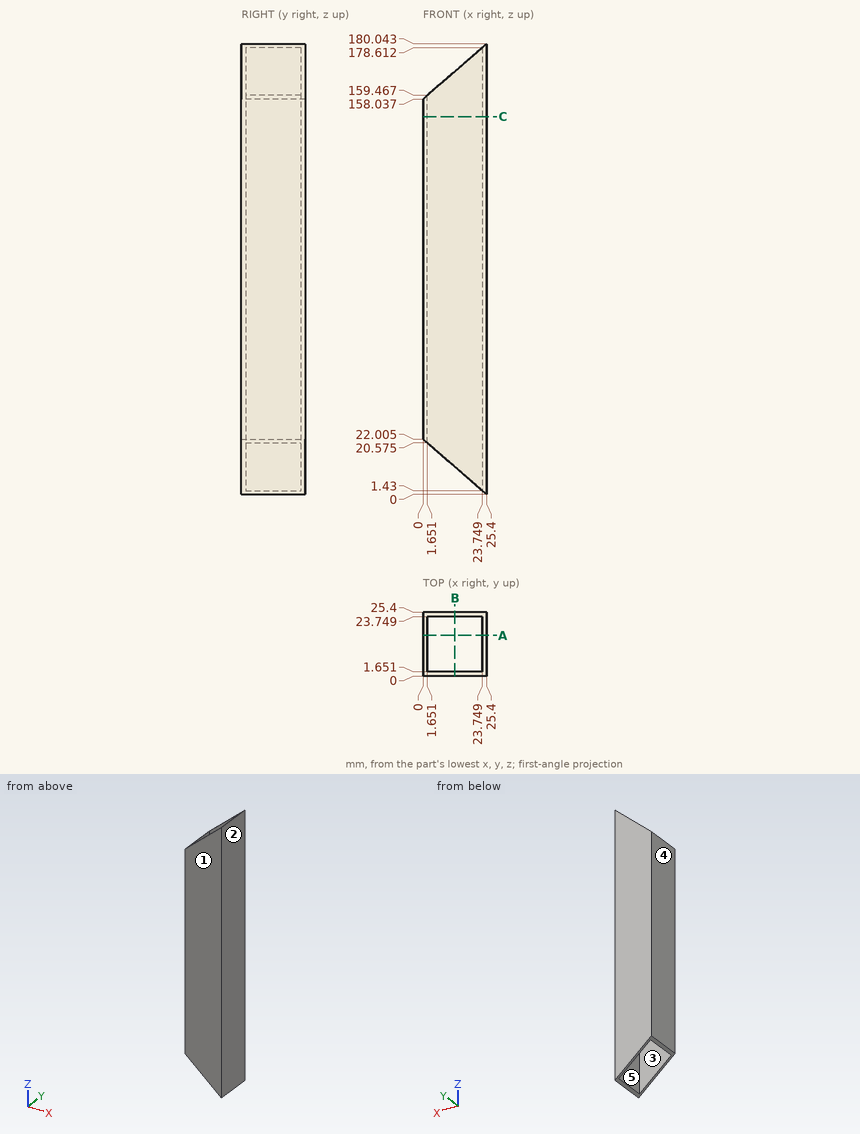
Study the drawing (mm; zero at the part's minimum x, y, z) and answer. A direction names the side the tool comes from. Round coordinates to 2 decimals unless told otherwise and drop trailing zeros. Write each loop counter-clockwise with the first axis right and the second up, starting at its lowest first coordinate (ties: lowest second). Pieces come first, ordered by that corner, then holes. Notation, with made-up numbers: (82, -30) -> (128, -30) arc R16 cw to (128, -10) -> close; hole circle Ø8 at (21, 53). An arc over 180 degrees is marked (long way). Answer as CSV lines item,"result". Start each with the question number.
(1) The part is cut by section C-C, the plane z = 151. Give the vertices of the cut face in (x, y).
(2) The part is cut by section A-A, the plane y = 16.25. Give the vertices of the cut face in (x, z) (1 decimal).
(3) A tool of negligible diameter and unlimited length cuts with its end or side. For the marked faces 4 and 5, from which of +Z, -Z, +X, -X, +Y, -Y can it reach the whole face along a straight path? Write none if from no direction.
(4) The part is cut by section B-B, the plane x = 12.75. Give the vertices of the cut face in (y, z).
(5) Find the intervals of material crossed by probe 1 along X at (y, z) = (22, 113); probe 2 along X at (y, z) = (15.75, 16), in increasing order.
(6) The mould has two halves that part along Y. Classify the marked faces 1, 2 and 3: +Y half, -Y half, draft (parallel to the pull), parting line (faces both ways), or undercut.
Output values:
1,outline,"(0, 0) -> (25.4, 0) -> (25.4, 25.4) -> (0, 25.4) -> close; hole (1.65, 1.65) -> (23.75, 1.65) -> (23.75, 23.75) -> (1.65, 23.75) -> close"
2,outline,"(0, 22) -> (1.7, 20.6) -> (1.7, 159.5) -> (0, 158) -> close; (23.7, 1.4) -> (25.4, 0) -> (25.4, 180) -> (23.7, 178.6) -> close"
3,face 4,"+Z, -Z, -X, +Y, -Y"
3,face 5,"+Z, -Z"
4,outline,"(0, 10.96) -> (1.65, 10.96) -> (1.65, 169.08) -> (0, 169.08) -> close; (23.75, 10.96) -> (25.4, 10.96) -> (25.4, 169.08) -> (23.75, 169.08) -> close"
5,probe 1,"x = 0 to 1.65, 23.75 to 25.4"
5,probe 2,"x = 23.75 to 25.4"
6,face 1,"-Y half"
6,face 2,"draft"
6,face 3,"undercut"
